from build123d import *

# Parameters (mm, degrees)
F0_R       = 1.25
F1_DEPTH   = 2
F0_W       = 50
F0_H       = 2
F2_DEPTH   = 15
F3_SIZE2   = 2.7474774195
F3_SIZE    = 1
F3_2_SIZE2 = 2.7474774195
F3_2_SIZE  = 1
F3_3_SIZE2 = 2.7474774195
F3_3_SIZE  = 1
F4_W       = 2.75
F4_H       = 1
F4_W_2     = 1
F4_H_2     = 2.75
F5_DEPTH   = 10
F6_W       = 2
F6_H       = 5
F7_DEPTH   = 8
F8_SIZE    = 4.99999


# Not quite as in the source:
# - a fillet or chamfer is up to 0.001 mm smaller than in the source, because OpenCascade refuses the exact size
# - a feature names something its author has since deleted; it is built from what else it names


with BuildPart() as f1:
    # F0 (on Top) → F1 (new body)
    with BuildSketch(Plane.XY):
        Polygon((-30, 5), (-65, 5), (-65, -5), (65, -5), (65, 5), (20, 5), (10, 5), (-20, 5), align=None)
        with Locations((-61, -1)):
            Circle(F0_R, mode=Mode.SUBTRACT)
        with Locations((60.2, -1)):
            Circle(F0_R, mode=Mode.SUBTRACT)
        with Locations((-61, -1)):
            Circle(F0_R)
        with Locations((60.2, -1)):
            Circle(F0_R)
        Polygon((-30, 114.35), (-30, 5), (-20, 5), (-20, 104.35), (10, 104.35), (10, 5), (20, 5), (20, 114.35), align=None)
    extrude(amount=F1_DEPTH)

    # F0 (on Top) → F2 (join)
    with BuildSketch(Plane.XY):
        with Locations((60.2, -1)):
            Circle(F0_R)
        with Locations((-61, -1)):
            Circle(F0_R)
        with Locations((-5, 115.35)):
            Rectangle(F0_W, F0_H)
    extrude(amount=F2_DEPTH)

    # F3
    f3_edges = [f1.edges().sort_by_distance(p)[0] for p in [
        (58.95, -1, 15),
    ]]
    f3_side = f1.faces().sort_by_distance((60.2, -1, 15))[0]
    chamfer(f3_edges, length=F3_SIZE, length2=F3_SIZE2, reference=f3_side)

    # F3#2
    f3_2_edges = [f1.edges().sort_by_distance(p)[0] for p in [
        (-62.25, -1, 15),
    ]]
    f3_2_side = f1.faces().sort_by_distance((-61, -1, 15))[0]
    chamfer(f3_2_edges, length=F3_2_SIZE, length2=F3_2_SIZE2, reference=f3_2_side)

    # F3#3
    f3_3_edges = [f1.edges().sort_by_distance(p)[0] for p in [
        (-5, 114.35, 15),
    ]]
    f3_3_side = f1.faces().sort_by_distance((-5, 115.35, 15))[0]
    chamfer(f3_3_edges, length=F3_3_SIZE, length2=F3_3_SIZE2, reference=f3_3_side)

    # F4 (on face) → F5 (join)
    with BuildSketch(Plane.XY.offset(2)):
        with Locations((-62.875, -1)):
            Rectangle(F4_W, F4_H)
        with Locations((-61, 0.875)):
            Rectangle(F4_W_2, F4_H_2)
        with Locations((-61, -1)):
            Rectangle(F4_W_2, F4_H)
        with Locations((-59.125, -1)):
            Rectangle(F4_W, F4_H)
        with Locations((-61, -2.875)):
            Rectangle(F4_W_2, F4_H_2)
        with Locations((60.2, 0.875)):
            Rectangle(F4_W_2, F4_H_2)
        with Locations((60.2, -1)):
            Rectangle(F4_W_2, F4_H)
        with Locations((58.325, -1)):
            Rectangle(F4_W, F4_H)
        with Locations((62.075, -1)):
            Rectangle(F4_W, F4_H)
        with Locations((60.2, -2.875)):
            Rectangle(F4_W_2, F4_H_2)
    extrude(amount=F5_DEPTH)

    # F6 (on face) → F7 (join)
    with BuildSketch(Plane.XY.offset(2)):
        with Locations((-19, 111.85)):
            Rectangle(F6_W, F6_H)
        with Locations((11, 111.85)):
            Rectangle(F6_W, F6_H)
    extrude(amount=F7_DEPTH)

    # F8 (size 5 in the source; OpenCascade refuses exactly that, so slightly less here)
    f8_edges = [f1.edges().sort_by_distance(p)[0] for p in [
        (-19, 109.35, 10),
        (11, 109.35, 10),
    ]]
    chamfer(f8_edges, length=F8_SIZE)


solid = f1.part
For this review, take the finished solid that the model builds, in its own axes (mm). A direction names the side the tool comes from. Give positions to 0.01 mm unless a question says otherwise; leave off trailing zeros. Order: outer loops, then holes, each group sorted by start corner. A loop starts at its lowest first (then second) coordinate and runs counter-clockwise, first axis right, second up. Notation, with made-up numbers: M 30,75.25 L 45,75.25 A35 cw 45,111.25 Z; hole C 72,71.25 d7. An arc over 180 degrees is marked long. Answer in a Markdown table with one row per item. Add a question column.
(1) For faces 4 (the face through (-30, 69, 1)), 5 (the face through (10, 112, 5)), 6 (the face through (-5, 116.35, 7)), 7 (the face through (20, 60, 1)), 8 (the face through (12, 112, 5)), list the 3-axis set-ups (+Z, -Z, +X, -X, +Y, -Y) from which the entire face can be reached by the end or side of a thin tool; tool diameter is ignored.
(2) Mouldability with a two-part tool opening along X and no side actions: class faces 1 (the face through (-20, 112, 5)), 2 (the face through (14, 51, 0)), 3 (the face through (-5, 114.35, 7)) as +X half, -X half, draft (parallel to the pull), parting line (faces both ways), or undercut.
(3) Consider section A-A on x = -15.5. State the section outline as (y, z) points.
(4) Consider section C-C on x = -35.5. State the section outline as (y, z) points, and give its area (3 significant figures).
(5) For pin 1 (5 mm diameter, centred on x = -28, y = 72, fed in from -Z); pin 2 (7.5 mm diameter, centred on y = 81, z = 5.5, fed in from +X); pin 3 (1.7 mm diameter, centred on y = -3.5, z = 9, fed in from -X); pin 4 (12 mm diameter, centred on x = 15, y = 91.5, fed in from +Z), all flat-tipped, find the tip position at first contact; note any pin that passes through.
(6) Consider section B-B on y = 20.5. State the section outline as (x, z) points, and give its area (3 significant figures).
(7) Wall thickness on probe 1 along Z at (x, y) = (-21.5, 43); probe 2 along Y at (x, z) = (-11.5, 4); probe 3 along X at (y, z) = (0, 3.75): over which ranges is each line inside the solid? List them lowest first. Write a range as [from, to].
Evaluation:
| question | item | result |
|---|---|---|
| 1 | face 4 | +Z, -Z, -X, +Y |
| 1 | face 5 | +Z, -Y |
| 1 | face 6 | +Z, -Z, +X, -X, +Y |
| 1 | face 7 | +Z, -Z, +X, +Y |
| 1 | face 8 | +Z, +X, -Y |
| 2 | face 1 | -X half |
| 2 | face 2 | draft |
| 2 | face 3 | undercut |
| 3 | outline | M -5,0 L 5,0 L 5,2 L -5,2 Z; M 104.35,0 L 116.35,0 L 116.35,15 L 115.35,15 L 114.35,12.25 L 114.35,2 L 104.35,2 Z |
| 4 | outline | M -5,0 L 5,0 L 5,2 L -5,2 Z |
| 4 | area | 20.0 mm^2 |
| 5 | pin 1 | stops at z = 0 |
| 5 | pin 2 | stops at x = 20 |
| 5 | pin 3 | stops at x = -61.5 |
| 5 | pin 4 | stops at z = 2 |
| 6 | outline | M -30,0 L -20,0 L -20,2 L -30,2 Z; M 10,0 L 20,0 L 20,2 L 10,2 Z |
| 6 | area | 40.0 mm^2 |
| 7 | probe 1 | z = [0, 2] |
| 7 | probe 2 | y = [114.35, 116.35] |
| 7 | probe 3 | x = [-61.75, -60.25], [59.45, 60.95] |
